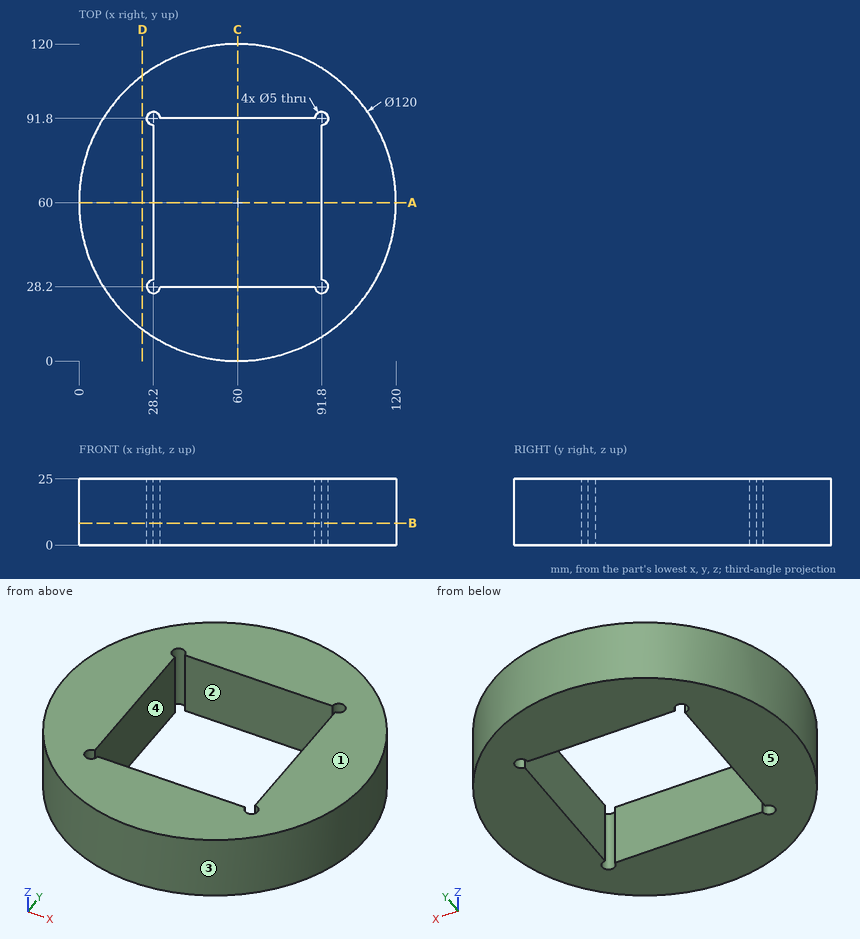
Input: dimensioned drawing with shaded views. Units: mm. Origin: part minimum x, y, z. A direction names the side the tool comes from. Coordinates: 2 decimals unless noted, no trailing zeros. Write each loop counter-clockwise with the first axis right and the second up, starting at its lowest first coordinate (ties: lowest second). Pieces come first, ordered by that corner, then holes. Notation, with made-up numbers: (86.5, 47.5) -> (91.5, 47.5) arc R26 cw to (91.5, 78.5) -> close; hole circle Ø3 at (28, -8.75). An arc over 180 degrees is marked (long way). Return JSON: item names as keys, results as strings. Group by question number.
1) Section query D-D, the plane x = 24. Return loops of the section in (y, z), plus the area to 3 significant figures.
2) Ray query, line 1 along X through (y, z) = (94, 10); line 2 along Y through (x, z) = (79, 23); line 3 along Y through (x, z) = (69.5, 15). Return the intervals inside material, ascending.
3) Section query B-B, the plane z = 8.25. Return loops of the section in (x, y), plus the area to 3 significant figures.
4) Section query A-A, the plane y = 60. Return loops of the section in (x, z), plus the area to 3 significant figures.
5) Set-up query: the marked faces 1 and 2. Return all of +Z, -Z, +X, -X, +Y, -Y with unobstructed straight access to the full face (end or side cutting, diameter ignored); none if empty.
6) Mould query, pull axis X, two halves, no side actions, for the marked faces 3, 4 and 5. Classes: +X half, -X half, draft (parallel to the pull), parting line (faces both ways), or undercut.
7) Contact query for flat-ended pins moving along their axis: P1, Ø7.5, axis at y = 74, z = 14, coming from the -X side; P2, Ø5, axis at x = 26.5, z = 8, coming from the +Y side; P3, Ø6, axis at x = 62.5, z = 8.5, coming from the +Y side. Output: stop coordinate, or through.
From the geometry:
{
 "1": {"outline": "(12, 0) -> (108, 0) -> (108, 25) -> (12, 25) -> close", "area": "2,400 mm²"},
 "2": {"line 1": "10.56 to 27.01, 29.39 to 90.61, 92.99 to 109.44", "line 2": "3.09 to 28.2, 91.8 to 116.91", "line 3": "0.76 to 28.2, 91.8 to 119.24"},
 "3": {"outline": "circle Ø120 at (60, 60); hole (28.2, 30.7) arc R2.5 ccw (long way) to (30.7, 28.2) -> (89.3, 28.2) arc R2.5 ccw (long way) to (91.8, 30.7) -> (91.8, 89.3) arc R2.5 ccw (long way) to (89.3, 91.8) -> (30.7, 91.8) arc R2.5 ccw (long way) to (28.2, 89.3) -> close", "area": "7,210 mm²"},
 "4": {"outline": "(0, 0) -> (28.2, 0) -> (28.2, 25) -> (0, 25) -> close; (91.8, 0) -> (120, 0) -> (120, 25) -> (91.8, 25) -> close", "area": "1,410 mm²"},
 "5": {"face 1": "+Z, +X, -X, +Y, -Y", "face 2": "+Z, -Z"},
 "6": {"face 3": "parting line", "face 4": "undercut", "face 5": "draft"},
 "7": {"P1": "x = 0.88", "P2": "y = 111.37", "P3": "y = 120"}
}
